Here's how the part is built. I have some questions about the finished solid (model axes, mm). Face numbers are marked on the shaded views. A direction names the side the tool comes from. Round coordinates to 2 decimals unless told otherwise and drop trailing zeros. Write each loop counter-clockwise with the first axis right and the second up, starting at its lowest first coordinate (ties: lowest second). Pieces come first, ordered by that corner, then holes. Notation, with made-up numbers: (81, 31) -> (114, 31) arc R26 ccw to (114, 51) -> close; hole circle Ø4 at (17.25, 26). An arc over 180 degrees is marked (long way). Answer in a Markdown table with one row per item.
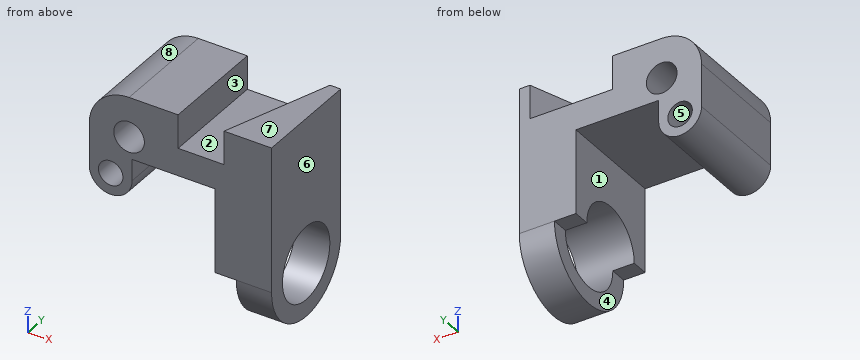
from build123d import *

# Parameters (mm, degrees)
F0_W     = 37
F0_H     = 55
F0_R     = 10
F1_DEPTH = 35
F3_DEPTH = 22
F4_W     = 23
F4_H     = 35
F6_R     = 24
F7_DEPTH = 37


with BuildPart() as f1:
    # F0 (on Front) → F1 (new body, symmetric)
    with BuildSketch(Plane.XZ):
        with Locations((46.500005, -42.603335)):
            Rectangle(F0_W, F0_H)
        with BuildLine():
            Line((28.000005, -15.103335), (65.000005, -15.103335))
            Line((65.000005, -15.103335), (65.000005, 24.896665))
            Line((65.000005, 24.896665), (-27.999995, 24.896665))
            ThreePointArc((-27.999995, 24.896665), (-46.384771, 17.281441), (-53.999995, -1.103335))
            Line((-53.999995, -1.103335), (-53.999995, -15.103335))
            Line((-53.999995, -15.103335), (-25.999995, -15.103335))
            Line((-25.999995, -15.103335), (28.000005, -15.103335))
        make_face()
        with Locations((-27.999995, -1.103335)):
            Circle(F0_R, mode=Mode.SUBTRACT)
        with BuildLine():
            Line((-25.999995, -29.103335), (-25.999995, -15.103335))
            Line((-25.999995, -15.103335), (-53.999995, -15.103335))
            Line((-53.999995, -15.103335), (-53.999995, -29.103335))
            Line((-53.999995, -29.103335), (-47.999995, -29.103335))
            ThreePointArc((-47.999995, -29.103335), (-39.999995, -21.103335), (-31.999995, -29.103335))
            Line((-31.999995, -29.103335), (-25.999995, -29.103335))
        make_face()
        with BuildLine():
            ThreePointArc((-53.999995, -29.103335), (-39.999995, -43.103335), (-25.999995, -29.103335))
            Line((-25.999995, -29.103335), (-31.999995, -29.103335))
            ThreePointArc((-31.999995, -29.103335), (-39.999995, -37.103335), (-47.999995, -29.103335))
            Line((-47.999995, -29.103335), (-53.999995, -29.103335))
        make_face()
    extrude(amount=F1_DEPTH, both=True)

    # F2 (on face) → F3 (cut)
    with BuildSketch(Plane.XY.offset(24.896665)):
        Polygon((58.000005, 35), (4.000005, 35), (4.000005, -35), (34.000005, -35), align=None)
    extrude(amount=-F3_DEPTH, mode=Mode.SUBTRACT)

    # F4 (on face) → F5 (revolve)
    with BuildSketch(Plane(origin=(0, 0, -70.103335), x_dir=(1, 0, 0), z_dir=(0, 0, -1))):
        with Locations((53.500005, 17.5)):
            Rectangle(F4_W, F4_H)
    revolve(axis=Axis((53.500005, 0, -70.103335), (1, 0, 0)))

    # F6 (on face) → F7 (cut)
    with BuildSketch(Plane.YZ.offset(65.000005)):
        with Locations((0, -70.103335)):
            Circle(F6_R)
    extrude(amount=-F7_DEPTH, mode=Mode.SUBTRACT)


solid = f1.part
1) For pin 1 (8 mm diameter, centred on x = 30, y = 5, fed in from +Z); pin 2 (5 mm diameter, centred on x = 10.5, y = -23, fed in from -Z); pin 3 (10.5 mm diameter, centred on y = -6.5, z = -90.5, fed in from -X), each with a flat end and sliding along its axis, tell me the tip position at first contact or that it passes through.
Response:
| item | result |
|---|---|
| pin 1 | stops at z = 2.9 |
| pin 2 | stops at z = -15.1 |
| pin 3 | stops at x = 42 |
2) Which directions (+Z, -Z, +X, -X, +Y, -Y) give clear straight access to the entire face, cutting with the end or side of a thin tool? Please do the marked faces 1, 2, 3 and 4.
Response:
| item | result |
|---|---|
| face 1 | -Z, +Y, -Y |
| face 2 | +Z, +Y |
| face 3 | +Z, +Y, -Y |
| face 4 | -Z, -X, +Y, -Y |
3) We'd pull the mould along X, two halves only. Please class the marked faces 5, 6, 7 and 8: +X half, -X half, draft (parallel to the pull), parting line (faces both ways), or undercut.
Response:
| item | result |
|---|---|
| face 5 | undercut |
| face 6 | +X half |
| face 7 | draft |
| face 8 | -X half |
4) I need wall thicknesses on line 1 (X direction, y = -17, z = -23); line 2 (X direction, y = -14.5, z = -33); line 3 (Z direction, x = 53, y = 0). Which ranges of each line are inside material? Lowest first, please. Write a range as [from, to].
Response:
| item | result |
|---|---|
| line 1 | x = [-54, -45.17], [-34.83, -26], [28, 65] |
| line 2 | x = [-53.45, -46.99], [-33.01, -26.55], [28, 65] |
| line 3 | z = [-105.1, -94.1], [-46.1, 24.9] |
5) I want a section at C-C, the plane x = 40. List the corners of the cut face in (y, z) for me, and give its area (3 significant figures).
Response:
| item | result |
|---|---|
| outline | (-35, -70.1) -> (-24, -70.1) arc R24 cw to (24, -70.1) -> (35, -70.1) -> (35, 2.9) -> (-17.5, 2.9) -> (-17.5, 24.9) -> (-35, 24.9) -> close |
| area | 4,590 mm^2 |
6) I want a section at B-B, the plane z = -64. List the corners of the cut face in (x, y) for me.
Response:
| item | result |
|---|---|
| outline | (28, -35) -> (65, -35) -> (65, -23.21) -> (28, -23.21) -> close; (28, 23.21) -> (65, 23.21) -> (65, 35) -> (28, 35) -> close |
7) I want a section at A-A, the plane y = 0. List the corners of the cut face in (x, z) for me.
Response:
| item | result |
|---|---|
| outline | (-54, -29.1) arc R14 ccw to (-26, -29.1) -> (-26, -15.1) -> (28, -15.1) -> (28, -46.1) -> (65, -46.1) -> (65, 24.9) -> (46, 24.9) -> (46, 2.9) -> (4, 2.9) -> (4, 24.9) -> (-28, 24.9) arc R26 ccw to (-54, -1.1) -> close; (42, -105.1) -> (65, -105.1) -> (65, -94.1) -> (42, -94.1) -> close; hole circle Ø16 at (-40, -29.1); hole circle Ø20 at (-28, -1.1) |
8) I want a section at D-D, the plane y = 30. List the corners of the cut face in (x, z) for me, and give its area (3 significant figures).
Response:
| item | result |
|---|---|
| outline | (-54, -29.1) arc R14 ccw to (-26, -29.1) -> (-26, -15.1) -> (28, -15.1) -> (28, -70.1) -> (42, -70.1) -> (42, -88.13) -> (65, -88.13) -> (65, 24.9) -> (56.29, 24.9) -> (56.29, 2.9) -> (4, 2.9) -> (4, 24.9) -> (-28, 24.9) arc R26 ccw to (-54, -1.1) -> close; hole circle Ø16 at (-40, -29.1); hole circle Ø20 at (-28, -1.1) |
| area | 6,100 mm^2 |
